Check sheet for the drawn part. Datum: minimum x, y, z corner. Units: mm. A direction names the side the tool comes from. Give positions to 0.01 mm unless a question says otherwise; leave off trailing zeros. Order: outer loops, then holes, each group sorted by start corner. A loop starts at its lowest first (then second) coordinate and runs counter-clockwise, first axis right, second up.
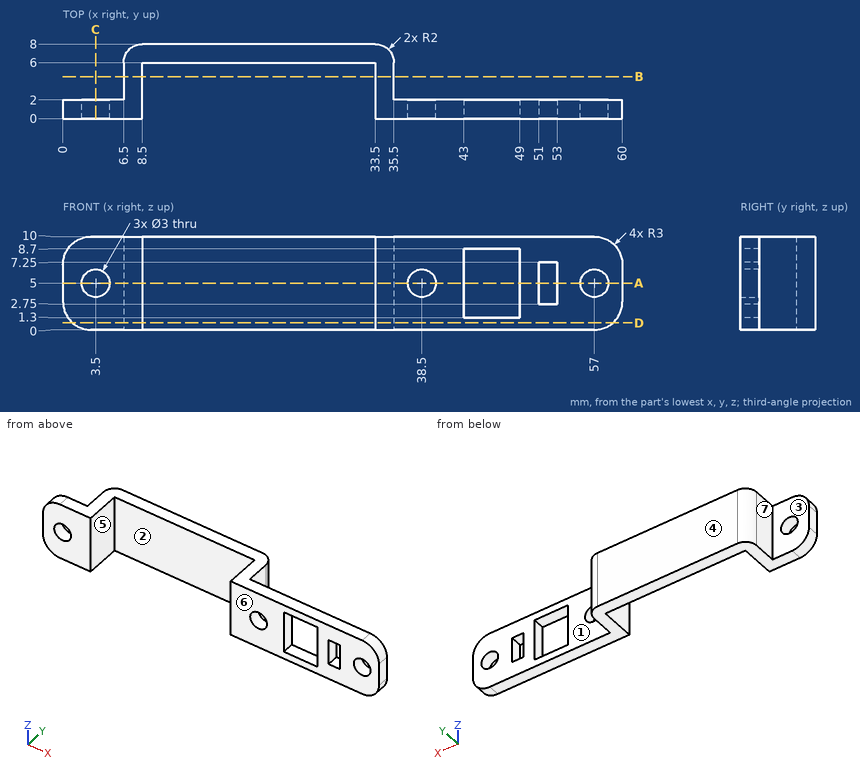
(1) Set-up check for the marked faces 1, 2, 3 and 4: record each of +Z, -Z, +X, -X, +Y, -Y from which the full face is reachable in a straight line by a thin tool's end or side.
Solved:
face 1: +Z, -Z, +X, +Y
face 2: +Z, -Z, -Y
face 3: +Z, -Z, -X, +Y
face 4: +Z, -Z, +X, -X, +Y
(2) Section check A-A, the plane z = 5. Give the number of separate pieces and of enclosed holes in the cut face, then the cut area to 3 significant figures.
Solved:
separate pieces: 6
enclosed holes: 0
area: 108 mm2
(3) Go/stop test with flat-tipped pins: pin 1 (4 mm diameter, centred on y = 4.5, z = 1.5, fed in from -X); pin 2 (3.5 mm diameter, centred on x = 57, z = 5, fed in from +Y); pin 3 (1.5 mm diameter, centred on x = 25.5, z = 1.5, fed in from -Y). Record where each tip stops, or that it passes through.
Solved:
pin 1: stops at x = 6.5
pin 2: stops at y = 2
pin 3: stops at y = 6
(4) Section check C-C, the plane x = 3.5. Enter the section's corners in (y, z).
Solved:
outline: (0, 0) - (2, 0) - (2, 3.5) - (0, 3.5) - close; (0, 6.5) - (2, 6.5) - (2, 10) - (0, 10) - close
(5) Section check B-B, the plane y = 4.5. Enter the section's corners in (x, z).
Solved:
outline: (6.5, 0) - (8.5, 0) - (8.5, 10) - (6.5, 10) - close; (33.5, 0) - (35.5, 0) - (35.5, 10) - (33.5, 10) - close
(6) Scan lines: line 1 (X direction, y = 1.25, z = 3); line 2 (Z direction, x = 38.5, y = 0.65); line 3 (X direction, y = 5.75, z = 5.75). Record each from-to range of solid material in increasing order.
Solved:
line 1: x = 0 to 8.5, 33.5 to 43, 49 to 51, 53 to 60
line 2: z = 0 to 3.5, 6.5 to 10
line 3: x = 6.5 to 8.5, 33.5 to 35.5
(7) Section check D-D, the plane z = 0.75. Enter the section's corners in (x, y), then the cut area to 3 significant figures.
Solved:
outline: (1.02, 0) - (8.5, 0) - (8.5, 6) - (33.5, 6) - (33.5, 0) - (58.98, 0) - (58.98, 2) - (35.5, 2) - (35.5, 6) arc R2 ccw to (33.5, 8) - (8.5, 8) arc R2 ccw to (6.5, 6) - (6.5, 2) - (1.02, 2) - close
area: 138 mm2
(8) Release check for a two-part mould opening along X. For the marked faces 5, 6 and 7 record: pulls with the +X half, pulls with the -X half, needs draft (parallel to the pull), parting line crosses it, or undercut.
Solved:
face 5: undercut
face 6: needs draft
face 7: pulls with the -X half
